Autodesk Inventor part; units mm, degrees
ref_plane "YZ Plane" through (0, 0, 0) normal (1, 0, 0) x (0, 1, 0)
ref_plane "XZ Plane" through (0, 0, 0) normal (0, 1, 0) x (-1, 0, 0)
ref_plane "XY Plane" through (0, 0, 0) normal (0, 0, 1) x (1, 0, 0)
sketch "Sketch1" plane through (0, 0, 0) normal (0, 1, 0) x (-1, 0, 0)
  line L0 (0, 0) -> (-42, 0)
  line L1 (-42, 0) -> (-42, -42)
  line L2 (-42, -42) -> (0, -42)
  line L3 (0, -42) -> (0, 0)
  dimension "d0" = 42
  dimension "d1" = 42
extrude "Extrusion1" add sketch "Sketch1" along normal blind 47.5
chamfer "Chamfer1" distance 5 angle 45 4 edges at (42, 23.75, 0) (0, 23.75, 0) (0, 23.75, -42) (42, 23.75, -42)
sketch "Sketch3" plane through (0, 47.5, 0) normal (0, 1, 0) x (1, 0, 0)
  line L0 (0, 0) -> (42, 0)
  line L1 (42, 0) -> (42, 42)
  line L2 (42, 42) -> (0, 42)
  line L3 (0, 42) -> (0, 0)
  line L4 (37, 42) -> (5, 42)
  line L5 (42, 5) -> (42, 37)
extrude "Extrusion2" add sketch "Sketch3" against normal blind 7
sketch "Sketch4" plane through (0, 0, 0) normal (0, -1, 0) x (1, 0, 0)
  line L0 (0, 0) -> (42, 0)
  line L1 (0, -42) -> (0, 0)
  line L2 (42, 0) -> (0, 0)
  line L3 (0, 0) -> (0, -42)
  line L4 (0, -42) -> (42, -42)
  line L5 (42, -42) -> (42, 0)
extrude "Extrusion3" add sketch "Sketch4" against normal blind 7
chamfer "Chamfer2" distance 2 angle 45 8 edges at (42, 44, 0) (42, 3.5, 0) (42, 44, -42) (42, 3.5, -42) (0, 3.5, -42) (0, 3.5, 0) (0, 44, 0) (0, 44, -42)
sketch "Sketch5" plane through (0, 0, 0) normal (0, -1, 0) x (1, 0, 0)
  circle A0 centre (21, -21) radius 5
  line L0 (40, -42) -> (2, -42)
  line L1 (42, -40) -> (42, -2)
  point P0 (0, 0)
  dimension "d14" = 10
  dimension "d15" = 21
  dimension "d16" = 21
extrude "Extrusion4" cut sketch "Sketch5" against normal blind 7
sketch "Sketch6" plane through (0, 47.5, 0) normal (0, 1, 0) x (1, 0, 0)
  circle A0 centre (21, 21) radius 5
  circle A1 centre (21, 21) radius 5
  circle A2 centre (21, 21) radius 11
  point P0 (0, 0)
  dimension "d19" = 10
  dimension "d20" = 22
extrude "Extrusion5" add sketch "Sketch6" along normal blind 2
sketch "Sketch7" plane through (0, 47.5, 0) normal (0, 1, 0) x (1, 0, 0)
  circle A0 centre (5.25, 5.25) radius 1.6
  circle A1 centre (5.25, 36.75) radius 1.6
  circle A2 centre (36.75, 36.75) radius 1.6
  circle A3 centre (36.75, 5.25) radius 1.6
  line L0 (2, 0) -> (40, 0)
  line L1 (0, 40) -> (0, 2)
  point P0 (0, 0)
  dimension "d23" = 3.2
  dimension "d24" = 3.2
  dimension "d25" = 3.2
  dimension "d26" = 3.2
  dimension "d27" = 31.5
  dimension "d28" = 31.5
  dimension "d29" = 31.5
  dimension "d30" = 31.5
  dimension "d31" = 5.25
  dimension "d32" = 5.25
  dimension "d33" = 5.25
  dimension "d34" = 5.25
extrude "Extrusion6" cut sketch "Sketch7" against normal blind 10
sketch "Sketch8" plane through (0, 0, 0) normal (0, -1, 0) x (1, 0, 0)
  circle A0 centre (5.25, -36.75) radius 1.6
  circle A1 centre (5.25, -36.75) radius 1.6
  circle A2 centre (5.25, -5.25) radius 1.6
  circle A3 centre (5.25, -5.25) radius 1.6
  circle A4 centre (36.75, -36.75) radius 1.6
  circle A5 centre (36.75, -36.75) radius 1.6
  circle A6 centre (36.75, -5.25) radius 1.6
  circle A7 centre (36.75, -5.25) radius 1.6
  point P0 (0, 0)
  dimension "d37" = 3.2
  dimension "d38" = 3.2
  dimension "d39" = 3.2
  dimension "d40" = 3.2
extrude "Extrusion7" cut sketch "Sketch8" against normal blind 2
sketch "Sketch9" plane through (21, 47.5, -21) normal (0, 1, 0) x (1, 0, 0)
  circle A0 centre (0, 0) radius 2.5
  line L0 (-21, 19) -> (-21, -19)
  line L1 (-19, -21) -> (19, -21)
  point P0 (-21, -21)
  dimension "d43" = 5
  dimension "d44" = 21
  dimension "d45" = 21
extrude "Extrusion8" add sketch "Sketch9" along normal blind 24
chamfer "Chamfer3" distance 1 angle 45 1 edges at (18.5, 71.5, -21)
properties part number "Nema17" material "Gold"
Build history of the part. All positions in model axes, mm. A direction names the side the tool comes from. Round coordinates to 2 decimals unless told otherwise and drop trailing zeros. Loops run counter-clockwise (first coordinate to the right, second up) from the corner with the lowest first, then second, coordinate; pieces in that order, holes last.
Item 1: Saw through at B-B (x = 21). List the corners of the cut face in (y, z), then the cut area to 3 significant figures.
Item 2: Drill centre lines: line 1 along Z through (x, y) = (36.75, 40.5); line 2 along X through (y, z) = (1, -5); line 3 along Y through (x, z) = (35, -30). Where is each one in solid material? Low to high.
Item 3: Pin check, flat tips, straight feed: P1, Ø2.5, axis at x = 36.75, z = -36.75, coming from the -Y side; P2, Ø2, axis at x = 9, y = 52, coming from the +Z side; P3, Ø5.5, axis at x = 3.5, z = -3.5, coming from the +Y side. Stop position of each tip, or through.
Item 4: Saw through at C-C (y = 11). List the corners of the cut face in (x, z), then the cut area to 3 significant figures.
Item 5: Which spindle directions (+Z, -Z, +X, -X, +Y, -Y) get a long thin tool onto all of the face, cutting with end or side? Do faces 1 (the face through (5, 2, -37)), 2 (the face through (18.5, 58.8, -20.9)), 3 (the face through (2, 40.5, -40)), 4 (the face through (2, 40.5, -2)), 5 (the face through (40, 40.5, -2)). Say none if no direction does.
Item 6: Saw through at D-D (x = 13). List the corners of the cut face in (y, z).
Item 7: Two-plate mould, pull along Z, no slides. Class faces 6 (the face through (1, 44, -1)), 7 (the face through (41, 4, -41)), 8 (the face through (23, 47.5, -19)), 9 (the face through (37, 37.5, -37)): released by +Z, released by -Z, zero draft, split by the parting line, or undercut.
Item 8: Saw through at A-A (z = -21). List the corners of the cut face in (x, y), then the cut area to 3 significant figures.
Worked answers:
1. outline: (0, -42) - (47.5, -42) - (47.5, -32) - (49.5, -32) - (49.5, -26) - (47.5, -26) - (47.5, -23.5) - (70.5, -23.5) - (71.5, -22.5) - (71.5, -19.5) - (70.5, -18.5) - (47.5, -18.5) - (47.5, -16) - (49.5, -16) - (49.5, -10) - (47.5, -10) - (47.5, 0) - (0, 0) - (0, -16) - (7, -16) - (7, -26) - (0, -26) - close
1. area: 2,070 mm2
2. line 1: z = -42 to -38.35, -35.15 to -6.85, -3.65 to 0
2. line 2: x = 0 to 3.67, 6.83 to 35.17, 38.33 to 42
2. line 3: y = 0 to 47.5
3. P1: stops at y = 2
3. P2: passes through
3. P3: stops at y = 47.5
4. outline: (0, -37) - (5, -42) - (37, -42) - (42, -37) - (42, -5) - (37, 0) - (5, 0) - (0, -5) - close
4. area: 1,710 mm2
5. face 1: -Y
5. face 2: +Y
5. face 3: -Z, -X
5. face 4: +Z, -X
5. face 5: +Z, +X
6. outline: (0, -42) - (47.5, -42) - (47.5, -28.55) - (49.5, -28.55) - (49.5, -13.45) - (47.5, -13.45) - (47.5, 0) - (0, 0) - close
7. face 6: released by +Z
7. face 7: released by -Z
7. face 8: undercut
7. face 9: undercut
8. outline: (0, 0) - (16, 0) - (16, 7) - (26, 7) - (26, 0) - (42, 0) - (42, 47.5) - (32, 47.5) - (32, 49.5) - (26, 49.5) - (26, 47.5) - (23.5, 47.5) - (23.5, 70.5) - (22.5, 71.5) - (19.5, 71.5) - (18.5, 70.5) - (18.5, 47.5) - (16, 47.5) - (16, 49.5) - (10, 49.5) - (10, 47.5) - (0, 47.5) - close
8. area: 2,070 mm2
